CAD build for the part. Positions are in the model's coordinates, mm. Face numbers are marked on the shaded views. A direction names the side the tool comes from. Give positions to 0.01 mm unless a question says otherwise; leave off trailing zeros. Loops run counter-clockwise (first coordinate to the right, second up) from the corner with the lowest first, then second, coordinate; pieces in that order, holes last.
```python
from build123d import *

# Parameters (mm, degrees)
EXTRUDE_1_DEPTH         = 215
EXTRUDE_2_DEPTH         = 1
EXTRUDE_3_DEPTH         = 1
SKETCH_4_W              = 246
SKETCH_4_H              = 137.991605588
CUT_EXTRUDE_1_DEPTH     = 333.555002245
CUT_EXTRUDE_2_REACH     = 274.801
SKETCH_5_W              = 74.6
SKETCH_5_H              = 83.6
FILLET_1_R              = 2
CUT_EXTRUDE_3_REACH     = 334.555
SKETCH_7_W              = 31
SKETCH_7_H              = 40
FILLET_2_R              = 2
FILLET_3_R              = 1
HOLE_WIZARD_M41_D       = 4.2
EXTRUDE_4_DEPTH         = 1
SKETCH_14_W             = 68
SKETCH_14_H             = 1
EXTRUDE_5_DEPTH         = 11
SKETCH_15_W             = 25
SKETCH_15_H             = 2
EXTRUDE_6_DEPTH         = 10
EXTRUDE_7_DEPTH         = 14
HOLE_WIZARD_M41_2_D     = 3.3
HOLE_WIZARD_M41_2_DEPTH = 1
HOLE_WIZARD_M42_D       = 3.3
HOLE_WIZARD_M42_DEPTH   = 2


with BuildPart() as part:
    # Эскиз1 → Бобышка-Вытянуть1 (new, symmetric)
    with BuildSketch(Plane(origin=(0, 0, 0), x_dir=(0, 0, -1), z_dir=(1, 0, 0))):
        Polygon((-97.817266744, 64), (-97.817266744, 0), (-96.817266744, 0), (-96.817266744, 63.385363703), (-42.261330955, 91), (42.278938578, 91), (137.622640037, 46.680562515), (137.622640037, 33.718332981), (106.182733256, 0.68946939), (106.907048077, 0), (138.622640037, 33.318481758), (138.622640037, 47.318481758), (42.5, 92), (-42.5, 92), align=None)
    extrude(amount=EXTRUDE_1_DEPTH, both=True)

    # Эскиз2 → Бобышка-Вытянуть2 (add)
    with BuildSketch(Plane(origin=(215, 0, 0), x_dir=(0, 0, -1), z_dir=(1, 0, 0))):
        Polygon((-96.817266744, 0), (-96.817266744, 63.385363703), (-42.261330955, 91), (42.278938578, 91), (137.622640037, 46.680562515), (137.622640037, 33.718332981), (105.526432948, 0), align=None)
    extrude(amount=-EXTRUDE_2_DEPTH)

    # Эскиз3 → Бобышка-Вытянуть3 (add)
    with BuildSketch(Plane.ZY.offset(215)):
        Polygon((96.817266744, 0), (96.817266744, 63.385363703), (42.261330955, 91), (-42.278938578, 91), (-137.622640037, 46.680562515), (-137.622640037, 33.718332981), (-105.526432948, 0), align=None)
    extrude(amount=-EXTRUDE_3_DEPTH)

    # Эскиз4 → Вырез-Вытянуть1 (cut, through all)
    with BuildSketch(Plane.XY.offset(97.817266744)):
        with Locations((32, 114.995802794)):
            Rectangle(SKETCH_4_W, SKETCH_4_H)
    extrude(amount=-CUT_EXTRUDE_1_DEPTH, mode=Mode.SUBTRACT)

    # Эскиз5 → Вырез-Вытянуть2 (cut, up to next)
    with BuildSketch(Plane(origin=(0, 91.898645501, -42.718042324), x_dir=(1, 0, 0), z_dir=(0, 0.9068173588352332, -0.42152375699964034)), mode=Mode.PRIVATE) as cut_extrude_2_sk1:
        with Locations((-153, 51.559552107)):
            Rectangle(SKETCH_5_W, SKETCH_5_H)
    cut_extrude_2_tool1 = extrude(cut_extrude_2_sk1.sketch, amount=-CUT_EXTRUDE_2_REACH, mode=Mode.PRIVATE) & part.part
    add(cut_extrude_2_tool1.solids().sort_by_distance((-153, 70.165069, -89.473139))[0], mode=Mode.SUBTRACT)

    # Скругление1
    fillet_1_edges = [part.edges().sort_by_distance(p)[0] for p in [
        (-115.7, 52.091967665, -127.167342908),
        (-115.7, 87.331353751, -51.35741171),
        (-190.3, 87.331353751, -51.35741171),
        (-190.3, 52.091967665, -127.167342908),
    ]]
    fillet(fillet_1_edges, radius=FILLET_1_R)

    # Эскиз7 → Вырез-Вытянуть3 (cut, up to next)
    with BuildSketch(Plane.XY.offset(97.817266744), mode=Mode.PRIVATE) as cut_extrude_3_sk1:
        with Locations((-177.5, 20)):
            Rectangle(SKETCH_7_W, SKETCH_7_H)
    cut_extrude_3_tool1 = extrude(cut_extrude_3_sk1.sketch, amount=-CUT_EXTRUDE_3_REACH, mode=Mode.PRIVATE) & part.part
    add(cut_extrude_3_tool1.solids().sort_by_distance((-177.5, 20, 97.817267))[0], mode=Mode.SUBTRACT)

    # Скругление2
    fillet_2_edges = [part.edges().sort_by_distance(p)[0] for p in [
        (-162, 0, 97.317266744),
        (-162, 40, 97.317266744),
        (-193, 40, 97.317266744),
        (-193, 0, 97.317266744),
    ]]
    fillet(fillet_2_edges, radius=FILLET_2_R)

    # Скругление3
    fillet_3_edges = [part.edges().sort_by_distance(p)[0] for p in [
        (-152.5, 91, -42.278938578),
        (-152.5, 91, 42.261330955),
        (-152.5, 63.385363703, 96.817266744),
        (185, 92, 42.5),
        (185, 92, -42.5),
        (0, 33.318481758, -138.622640037),
        (185, 64, 97.817266744),
        (184.5, 46.680562515, -137.622640037),
        (184.5, 91, -42.278938578),
        (184.5, 91, 42.261330955),
        (184.5, 63.385363703, 96.817266744),
        (-153, 92, 42.5),
        (-153, 92, -42.5),
        (-153, 47.318481758, -138.622640037),
        (-153, 64, 97.817266744),
    ]]
    fillet(fillet_3_edges, radius=FILLET_3_R)

    # Hole Wizard M41 (through all)
    with Locations(Plane.ZY.offset(215)):
        with Locations((72.817266744, 12), (-82.182733256, 12)):
            Hole(HOLE_WIZARD_M41_D / 2)

    # Эскиз13 → Бобышка-Вытянуть4 (add)
    with BuildSketch(Plane(origin=(-91, 0, 0), x_dir=(0, 0, -1), z_dir=(1, 0, 0))):
        with BuildLine():
            Line((137.622640037, 45), (137.622640037, 46.680562515))
            Line((137.622640037, 46.680562515), (42.278938578, 91))
            Line((42.278938578, 91), (-42.261330955, 91))
            Line((-42.261330955, 91), (-96.817266744, 63.385363703))
            Line((-96.817266744, 63.385363703), (-96.817266744, 53))
            Line((-96.817266744, 53), (-38.817266744, 53))
            Line((-38.817266744, 53), (-38.817266744, 69))
            ThreePointArc((-38.817266744, 69), (-34.130975243, 80.313708499), (-22.817266744, 85))
            Line((-22.817266744, 85), (36.622640037, 85))
            ThreePointArc((36.622640037, 85), (47.936348536, 80.313708499), (52.622640037, 69))
            Line((52.622640037, 69), (52.622640037, 45))
            Line((52.622640037, 45), (137.622640037, 45))
        make_face()
    extrude_4 = extrude(amount=-EXTRUDE_4_DEPTH)

    # Эскиз14 → Бобышка-Вытянуть5 (add)
    with BuildSketch(Plane(origin=(-91, 0, 0), x_dir=(0, 0, -1), z_dir=(1, 0, 0))):
        with Locations((86.622640037, 45.5)):
            Rectangle(SKETCH_14_W, SKETCH_14_H)
    extrude_5 = extrude(amount=EXTRUDE_5_DEPTH)

    # Эскиз15 → Бобышка-Вытянуть6 (add)
    with BuildSketch(Plane(origin=(-91, 0, 0), x_dir=(0, 0, -1), z_dir=(1, 0, 0))):
        with Locations((0.008803811, 90)):
            Rectangle(SKETCH_15_W, SKETCH_15_H)
    extrude_6 = extrude(amount=EXTRUDE_6_DEPTH)

    # Эскиз16 → Бобышка-Вытянуть7 (add)
    with BuildSketch(Plane(origin=(-91, 0, 0), x_dir=(0, 0, -1), z_dir=(1, 0, 0))):
        Polygon((-52.529527952, 54.51763809), (-48.906061321, 68.040599658), (-46.974209668, 67.522961568), (-50.5976763, 54), align=None)
    extrude_7 = extrude(amount=EXTRUDE_7_DEPTH)

    # Зеркальное отражение1: Бобышка-Вытянуть4, Бобышка-Вытянуть5, Бобышка-Вытянуть6, Бобышка-Вытянуть7 across plane
    add(extrude_4.mirror(Plane(origin=(32, 0, 0), x_dir=(0, 0, 1), z_dir=(1, 0, 0))))
    add(extrude_5.mirror(Plane(origin=(32, 0, 0), x_dir=(0, 0, 1), z_dir=(1, 0, 0))))
    add(extrude_6.mirror(Plane(origin=(32, 0, 0), x_dir=(0, 0, 1), z_dir=(1, 0, 0))))
    add(extrude_7.mirror(Plane(origin=(32, 0, 0), x_dir=(0, 0, 1), z_dir=(1, 0, 0))))

    # Hole Wizard M41 2
    with Locations(Plane(origin=(0, 0, -138.622640037), x_dir=(-1, 0, 0), z_dir=(0, 0, -1))):
        with Locations((-150.5, 41), (86.5, 41)):
            Hole(HOLE_WIZARD_M41_2_D / 2, depth=HOLE_WIZARD_M41_2_DEPTH)

    # Отверстие обработанное метчиком M42
    with Locations(Plane(origin=(0, 16.784371263, 62.640126326), x_dir=(1, 0, 0), z_dir=(0, 0.2588190451025141, 0.9659258262890702))):
        with Locations((-82.5, 46.563730151), (146.5, 46.563730151)):
            Hole(HOLE_WIZARD_M42_D / 2, depth=HOLE_WIZARD_M42_DEPTH)


solid = part.part
```
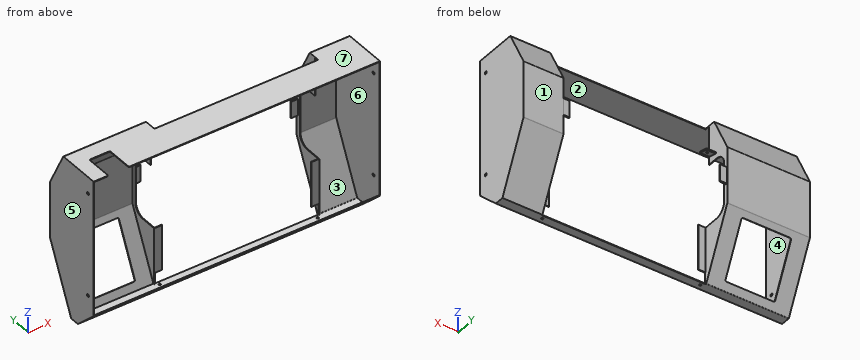
1. Saw through at A-A, the plane x = -147. List the corners of the cut face in (y, z), and give its area (3 significant figures).
Responses:
outline: (0, -106.91) - (33.03, -138.35) arc R1 ccw to (33.72, -138.62) - (46.68, -138.62) arc R1 ccw to (47.59, -138.04) - (52.55, -127.38) - (51.64, -126.96) - (46.68, -137.62) - (33.72, -137.62) - (0.69, -106.18) - close; (0, 96.82) - (62.77, 96.82) arc R1 cw to (63.66, 96.27) - (90.89, 42.47) arc R1 cw to (91, 42.02) - (91, -42.06) arc R1 cw to (90.91, -42.48) - (86.88, -51.15) - (87.78, -51.57) - (91.91, -42.7) arc R1 ccw to (92, -42.28) - (92, 42.26) arc R1 ccw to (91.89, 42.71) - (64.28, 97.27) arc R1 ccw to (63.39, 97.82) - (0, 97.82) - close
area: 291 mm2
2. Saw through at D-D, the plane x = 19.5. List the corners of the cut face in (y, z), and give its area (3 significant figures).
Responses:
outline: (0, -106.91) - (33.03, -138.35) arc R1 ccw to (33.72, -138.62) - (46, -138.62) - (46, -137.62) - (33.72, -137.62) - (0.69, -106.18) - close; (0, 96.82) - (46, 96.82) - (46, 97.82) - (0, 97.82) - close
area: 104 mm2
3. Probe line 1 along X through (y, z) = (49.5, -53); line 2 along Z through (x, y) = (161, 41); line 3 along X through (y, z) = (51.5, -17.5). List the from-to ranges inside material, lowest first.
Responses:
line 1: x = -215 to -214, -92 to -91, 155 to 156, 214 to 215
line 2: z = -138.62 to -137.62, 96.82 to 97.82
line 3: x = -215 to -214, 214 to 215
4. Drop flat-ended pins along their axis: pin 1 (0.5 mm diameter, centred on x = 155.5, z = -16, fed in from -Y); pin 2 (1.6 mm diameter, centred on x = 152.5, y = 90, fed in from -Z); pin 3 (3.5 mm diameter, centred on x = -85, y = 55, fed in from +Z). Give the stop position or say it passes through.
Responses:
pin 1: stops at y = 85
pin 2: stops at z = -12.51
pin 3: stops at z = 52.53
5. Tool access for the marked faces 1, 2 and 3: list every direction of +Z, -Z, +X, -X, +Y, -Y with a clear straight run to the whole face (end or side of a thin tool).
Responses:
face 1: +Z, -Z, +X, -X, +Y
face 2: -Y
face 3: none
6. Saw through at B-B, the plane z = 82.5. List the corners of the cut face in (x, y), and give its area (3 significant figures).
Responses:
outline: (-215, 0) - (-214, 0) - (-214, 70.63) - (-92, 70.63) - (-92, 53) - (-91, 53) - (-91, 71.75) - (-215, 71.75) - close; (155, 53) - (156, 53) - (156, 70.63) - (214, 70.63) - (214, 0) - (215, 0) - (215, 71.75) - (155, 71.75) - close
area: 383 mm2
7. Pull direction X, two halves, no side cores. Call the marked faces 4, 5, 6 and 7: released by +X, released by -X, zero draft, split by the parting line, or undercut.
Responses:
face 4: undercut
face 5: released by -X
face 6: undercut
face 7: zero draft
8. Saw through at C-C, the plane y = 19. List the corners of the cut face in (x, z).
Responses:
outline: (-215, -124.99) - (215, -124.99) - (215, 97.82) - (-162, 97.82) - (-162, 96.82) - (214, 96.82) - (214, -123.61) - (-214, -123.61) - (-214, 96.82) - (-193, 96.82) - (-193, 97.82) - (-215, 97.82) - close
